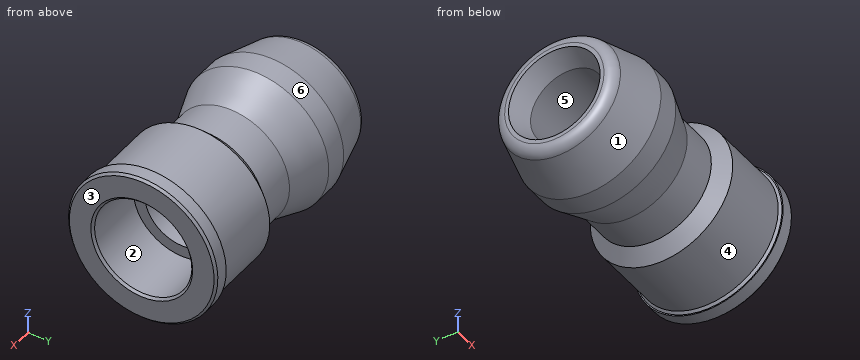
from build123d import *

# Parameters (mm, degrees)
M4_TAPPED_HOLE1_D           = 3.3
M4_TAPPED_HOLE1_CSINK_D     = 4.05
M4_TAPPED_HOLE1_CSINK_ANGLE = 45
FILLET1_R                   = 0.5
CHAMFER1_SIZE               = 0.1


with BuildPart() as part:
    # Sketch1 → Revolve1 (revolve)
    with BuildSketch(Plane.XY, mode=Mode.PRIVATE) as revolve1_sk:
        Polygon((5.889590125, 0), (0, 0), (0, 2.58), (2.3, 3.196283143), (3.3, 3.196283143), (5, 2.58), (6.62, 2.58), (7.19, 3.15), (10.34, 3.15), (10.34, 3.3), (11, 3.3), (11, 2.15), (8.3, 2.15), (8.3, 0), align=None)
    revolve(revolve1_sk.sketch.rotate(Axis((5.889590125, 0, 0), (-1, 0, 0)), 90), axis=Axis((5.889590125, 0, 0), (-1, 0, 0)))

    # M4 Tapped Hole1 (through all)
    with Locations(Plane.ZY):
        with Locations((0, 0)):
            CounterSinkHole(M4_TAPPED_HOLE1_D / 2, M4_TAPPED_HOLE1_CSINK_D / 2, counter_sink_angle=M4_TAPPED_HOLE1_CSINK_ANGLE)

    # Fillet1
    fillet1_edges = [part.edges().sort_by_distance(p)[0] for p in [
        (0, 0, 2.58),
    ]]
    fillet(fillet1_edges, radius=FILLET1_R)

    # Chamfer1
    chamfer1_edges = [part.edges().sort_by_distance(p)[0] for p in [
        (11, 0, 2.15),
        (11, 0, 3.3),
        (10.34, 0, 3.15),
    ]]
    chamfer(chamfer1_edges, length=CHAMFER1_SIZE)


solid = part.part
Design review of the part built by this model. Coordinates are the model's own, in mm. Face numbers are marked on the shaded views. A direction names the side the tool comes from. Coordinates: 2 decimals unless noted, no trailing zeros. Loops run counter-clockwise (first coordinate to the right, second up) from the corner with the lowest first, then second, coordinate; pieces in that order, holes last. Notation, with made-up numbers: (-19, 33) -> (30, 33) arc R16 ccw to (30, 59) -> close; hole circle Ø2 at (28.5, 29.5). An arc over 180 degrees is marked (long way). Use a Markdown table: item, result. Add a question column.
Item 1: We need section B-B, the plane x = 8.75. Write out the cut boundary in (y, z), and give its area (3 significant figures).
Item 2: Machinability: for the marked faces 4, 5 and 6, which of the approach directions +Z, -Z, +X, -X, +Y, -Y give a long, thin tool a straight path to every point of the face, cutting with its end or side? Answer none if there is none.
Item 3: We need section A-A, the plane x = 5.25. Write out the cut boundary in (y, z), and give its area (3 significant figures).
Item 4: Wall thickness on L1, parallel to Y at x = 6.25, z = 0; L2, parallel to Z at x = 4.5, y = 0.25; L3, parallel to Y at x = 7.25, z = 0: over which ranges is each line inside the solid? List them lowest first. Write a range as from..to.
Item 5: The part is to be moulded in two halves that separate along Y. For the marked faces 1, 2 and 3, say which applies: +Y half, -Y half, draft (parallel to the pull), parting line (faces both ways), or undercut.
Item 6: Clearance check with flat-ended pins moving along their axes: P1, Ø1, axis at y = 0.5, z = 1.5, coming from the +X side; P2, Ø2, axis at x = 7, z = 2, coming from the +Y side; P3, Ø1.5, axis at x = 7, z = 1.5, coming from the -Y side. State where each tip first meets the part, or that it passes through.
Numbers:
| question | item | result |
|---|---|---|
| 1 | outline | circle Ø6.3 at (0, 0); hole circle Ø4.3 at (0, 0) |
| 1 | area | 16.7 mm^2 |
| 2 | face 4 | none |
| 2 | face 5 | +X, -X |
| 2 | face 6 | -X |
| 3 | outline | circle Ø5.16 at (0, 0); hole circle Ø3.3 at (0, 0) |
| 3 | area | 12.4 mm^2 |
| 4 | L1 | y = -2.58..-1.65, 1.65..2.58 |
| 4 | L2 | z = -2.75..-1.63, 1.63..2.75 |
| 4 | L3 | y = -3.15..-1.65, 1.65..3.15 |
| 5 | face 1 | parting line |
| 5 | face 2 | undercut |
| 5 | face 3 | draft |
| 6 | P1 | stops at x = 8.3 |
| 6 | P2 | stops at y = 2.98 |
| 6 | P3 | stops at y = -3.05 |
